Autodesk Inventor part; units mm, degrees
ref_plane "Work Plane1" through (29, 0, 0) normal (0, -1, 0) x (1, 0, 0)
ref_plane "YZ Plane" through (0, 0, 0) normal (1, 0, 0) x (0, 1, 0)
ref_plane "XZ Plane" through (0, 0, 0) normal (0, 1, 0) x (-1, 0, 0)
sketch "Sketch1" plane through (0, 0, 0) normal (0, 0, 1) x (1, 0, 0)
  line L0 (0.0423, 0) -> (12.7, 0)
  line L1 (12.7, 0) -> (12.7, 3.9687)
  line L2 (12.7, 3.9687) -> (2.8196, 3.9687)
  line L3 (2.8196, 3.9687) -> (0.0001, 3.9688)
  line L4 (0.0001, 3.9688) -> (0, 3.9688)
  line L5 (0, 3.9688) -> (0, 6.9469)
  line L6 (0, 6.9469) -> (-4.2164, 6.9469)
  line L7 (-4.2164, 6.9469) -> (-4.2164, 2.757)
  line L8 (-4.2164, 2.757) -> (-1.5494, 2.757)
  line L9 (-1.5494, 2.757) -> (0.0423, 0)
  line L10 (-7.5997, 0) -> (16.0833, 0)
  line L11 (0, -1.3894) -> (0, 8.3363)
  line L12 (2.8196, 3.9687) -> (0, 3.9687) construction
  dimension "d1" = 9.8804
  dimension "d2" = 2.8195
  dimension "d3" = 4.2164
  dimension "d4" = 2.667
  dimension "d5" = 60
  dimension "d6" = 7.9375
  dimension "d7" = 7.9375
  dimension "d8" = 5.5139
  dimension "d9" = 13.8938
  dimension "d26" = 12.7
revolve "Body" add sketch "Sketch1" angle 360 about axis through (0.0423, 0, 0) along (1, 0, 0) contours L9 L11 L3 L2 L1 L0 | L9 L8 L7 L6 L5 L11
sketch "Sketch2" plane through (-4.2164, 0, 0) normal (-1, 0, 0) x (0, 0, 1)
  circle A0 centre (0, 0) radius 2.757
  line L0 (0, -9.7257) -> (0, 9.7257)
  line L1 (-9.7257, 0) -> (9.7257, 0)
  line L2 (2.757, 0) -> (1.3785, -2.3876)
  line L3 (1.3785, -2.3876) -> (-1.3785, -2.3876)
  line L4 (-1.3785, -2.3876) -> (-2.757, 0)
  line L5 (-2.757, 0) -> (-1.3785, 2.3876)
  line L6 (-1.3785, 2.3876) -> (1.3785, 2.3876)
  line L7 (1.3785, 2.3876) -> (2.757, 0)
extrude "Slot" add sketch "Sketch2" against normal up to next contours L7 A0 | A0 L2 | L6 L0 A0 | A0 L0 L3 | L0 L6 A0 | A0 L3 L0 | L4 A0 | A0 L5
fillet "Fillet1" radius 3.8354 1 edges at (-4.2164, -6.9469, 0)
thread "Thread"
chamfer "Chamfer1" distance 0.8656 distance2 0.8656 1 edges at (12.7, -3.9687, 0) measured on face at (12.7, -1.1714, -0.6148)
ref_plane "Work Plane1" through (29, 0, 0) normal (0, -1, 0) x (1, 0, 0)
fillet "Fillet2" radius 0.1 1 edges at (0.0001, -3.9688, 0)
equation "\"d1\" = GEL"
equation "\"d3\" = KOH"
equation "\"d4\" = INTI"
equation "\"d6\" = GD"
equation "\"d7\" = BDM"
equation "\"d8\" = 1.1547 * SW"
equation "\"d9\" = KOD"
equation "\"d26\" = NLG"
equation "\"d30\" = R"
equation "\"d17\" = RR"
equation "\"d13\" = GEL"
equation "\"d15\" = -0.5 * SPD + 0.5 * GD"
equation "\"d16\" = GUL"
equation "\"GD\" = NND"
equation "\"NLG\" = 12.7"
equation "\"GEL\" = 9.8804"
equation "\"KOD\" = 13.8938"
equation "\"KOH\" = 4.2164"
equation "\"INTI\" = 2.667"
equation "\"GAL\" = 2.8194"
equation "\"GUL\" = 0.86563"
equation "\"BDM\" = NND"
equation "\"SW\" = 4.7752"
equation "\"RR\" = 3.8354"
equation "\"SPD\" = 6.20624"
equation "\"R\" = 0.1"
equation "\"TOA\" = 30deg"
equation "\"GD1\" = SPD"
equation "\"THREADDIA\" = 7.9375"
equation "\"KOH1\" = 0.7874"
equation "\"NND\" = 7.9375"
equation "\"E0\" = 5.51536"
properties part number "ANSI B18.3 - 5/16 - 18 x 1/2" material "Steel, Mild"
Could you check a few things on this model? Use its own coordinates, in mm. A direction names the side the tool comes from. Round coordinates to 2 decimals unless told otherwise and drop trailing zeros. Loops run counter-clockwise (first coordinate to the right, second up) from the corner with the lowest first, then second, coordinate; pieces in that order, holes last. Notation, with made-up numbers: (-10, 0) - (11, 0) arc R26 ccw to (11, 32) - close; hole circle Ø7 at (34.25, 83.25). An arc over 180 degrees is marked (long way). Write item = value, one per line.
1) On a 3-axis mill with a long thin cutter (end or side, diameter ignored), from which of +Z, -Z, +X, -X, +Y, -Y can I reach the whole of each face in a straight line? I mean faces 4 (the conical face through (0, 4.1, -1.3)), 5 (the cylindrical face through (-0.19, -1.51, 6.78)), 6 (the flat face through (-3, -2.388, 0)). Say none if no direction works.
Computed:
face_4 = +X
face_5 = +X, -X
face_6 = -X
2) I need wall thicknesses on line 1 along Z through (x, y) = (-3, 2) (3 decimals); line 2 along Y through (x, z) = (3, -3.5); line 3 along Y through (x, z) = (2, 0.25). Which ranges of each line are inside material? Lowest first, please. Write a range as from..to.
Computed:
line_1 = -5.565..-1.602, 1.602..5.565
line_2 = -1.87..1.87
line_3 = -3.96..3.96
3) If we mould it in two halves opening along Z, with no side actions, what happens to faces 1 (the cylindrical face through (5.885, -0.86, 3.874)), 2 (the flat face through (-2.8, 1.21, 2.06)), 3 (the flat face through (12.7, 0, 0))? For each: pulls with the +Z half, pulls with the -Z half, needs draft (parallel to the pull), parting line crosses it, or undercut.
Computed:
face_1 = parting line crosses it
face_2 = undercut
face_3 = needs draft
4) Imagine slicing it at A-A (x = 0.75). Please give me the cut outline in (y, z).
Computed:
outline = circle Ø7.94 at (0, 0)
5) I'm going to push flat-ended pins straight in: P1, Ø0.8, axis at x = -3, z = 0, coming from the -Y side; P2, Ø3, axis at x = 2, y = 0, coming from the +Z side; P3, Ø4, axis at x = 2.5, z = -1, coming from the -Y side. Where does each tip first touch, or does it pass through?
Computed:
P1 = -6.24
P2 = 3.97
P3 = -3.97
